Can you work these out from the model? Positions are in its coordinate system, mm. A direction names the side the tool comes from. Round coordinates to 2 decimals unless told otherwise and drop trailing zeros. Loops run counter-clockwise (first coordinate to the right, second up) from the corner with the lowest first, then second, coordinate; pieces in that order, holes last. Notation, with made-up numbers: M 54.5,12.25 L 76.5,12.25 A25 ccw 76.5,25.25 Z; hole C 65,62 d2. An arc over 180 degrees is marked long. Return JSON: item names as keys, results as strings.
```python
from build123d import *

# Parameters (mm, degrees)
SKETCH1_W                       = 254
SKETCH1_H                       = 1016
BOSS_EXTRUDE1_DEPTH             = 203.2
FILLET1_RADIUS                  = 101.6
FILLET1_LENGTH                  = 254
BOSS_EXTRUDE2_DEPTH             = 25.4
BOSS_EXTRUDE2_DEPTH_BACK        = 279.4
SKETCH2_R                       = 12.7
CUT_EXTRUDE1_DEPTH              = 195.834
CUT_EXTRUDE1_DEPTH_BACK         = 440.182
SKETCH4_R                       = 12.7
BOSS_EXTRUDE3_REACH             = 1060.604
SKETCH5_W                       = 660.4
SKETCH5_H                       = 254
BOSS_EXTRUDE3_DIRECTION_2_REACH = 1060.604


with BuildPart() as part:
    # Sketch1 → Boss-Extrude1 (new body)
    with BuildSketch(Plane.XY):
        with Locations((127, 508)):
            Rectangle(SKETCH1_W, SKETCH1_H)
    extrude(amount=BOSS_EXTRUDE1_DEPTH)

    # Fillet1: full round fillet: the end face becomes a half cylinder, R = half its width
    fillet1_face = Plane((127, 0, 101.6), x_dir=(1, 0, 0), z_dir=(0, -1, 0))  # on the end face: x along it, z out of the body
    fillet1_slab = fillet1_face.offset(-FILLET1_RADIUS / 2) * Box(FILLET1_LENGTH, 2 * FILLET1_RADIUS, FILLET1_RADIUS, mode=Mode.PRIVATE)  # the body's end, R deep
    fillet1_round = Plane((127, 101.6, 101.6), x_dir=(0, -1, 0), z_dir=(1, 0, 0)) * Cylinder(FILLET1_RADIUS, FILLET1_LENGTH, mode=Mode.PRIVATE)  # its axis R under the face
    add(fillet1_slab - fillet1_round, mode=Mode.SUBTRACT)

    # Sketch2 → Boss-Extrude2 (add, two sides: drawn at the far end of the back side and taken through both)
    with BuildSketch(Plane(origin=(254, 0, 0), x_dir=(0, 0, -1), z_dir=(1, 0, 0)).offset(-BOSS_EXTRUDE2_DEPTH_BACK)):
        with Locations((-101.6, 25.4)):
            Circle(SKETCH2_R)
    extrude(amount=BOSS_EXTRUDE2_DEPTH + BOSS_EXTRUDE2_DEPTH_BACK)

    # Sketch4 → Cut-Extrude1 (cut, two sides: drawn at the far end of the back side and taken through both)
    with BuildSketch(Plane(origin=(254, 0, 0), x_dir=(0, 0, -1), z_dir=(1, 0, 0)).offset(-CUT_EXTRUDE1_DEPTH_BACK)):
        with Locations(Location((-101.6, 482.6, 0), (0, 0, 180))):
            Circle(SKETCH4_R)
    extrude(amount=CUT_EXTRUDE1_DEPTH + CUT_EXTRUDE1_DEPTH_BACK, mode=Mode.SUBTRACT)

    # Boss-Extrude3: up to this face of the body (flat: up to its plane)
    boss_extrude3_end = Plane(part.part.faces().sort_by_distance((127, 558.8, 203.2))[0])
    # Sketch5 → Boss-Extrude3 (add, up to the picked face)
    with BuildSketch(Plane.XY.offset(101.6), mode=Mode.PRIVATE) as boss_extrude3_sk1:
        with Locations((127, 889)):
            Rectangle(SKETCH5_W, SKETCH5_H)
    boss_extrude3_tool1 = split(extrude(boss_extrude3_sk1.sketch, amount=BOSS_EXTRUDE3_REACH, mode=Mode.PRIVATE), bisect_by=boss_extrude3_end, keep=Keep.BOTH, mode=Mode.PRIVATE)
    add(boss_extrude3_tool1.solids().sort_by(Axis((127, 889, 101.6), (0, 0, 1)))[0])

    # Boss-Extrude3 direction 2: up to this face of the body (flat: up to its plane)
    boss_extrude3_direction_2_end = Plane(part.part.faces().sort_by_distance((127, 558.8, 0))[0])
    # Sketch5 → Boss-Extrude3 direction 2 (add, up to the picked face)
    with BuildSketch(Plane.XY.offset(101.6), mode=Mode.PRIVATE) as boss_extrude3_direction_2_sk1:
        with Locations((127, 889)):
            Rectangle(SKETCH5_W, SKETCH5_H)
    boss_extrude3_direction_2_tool1 = split(extrude(boss_extrude3_direction_2_sk1.sketch, amount=-BOSS_EXTRUDE3_DIRECTION_2_REACH, mode=Mode.PRIVATE), bisect_by=boss_extrude3_direction_2_end, keep=Keep.BOTH, mode=Mode.PRIVATE)
    add(boss_extrude3_direction_2_tool1.solids().sort_by(Axis((127, 889, 101.6), (0, 0, -1)))[0])


solid = part.part
```
Q1. Suppose I cut it at C-C, the plane x = 83. Please give me the cut outline in (y, z), plus the area to 3 significant figures.
Results:
{"outline": "M 101.6,0 L 1016,0 L 1016,203.2 L 101.6,203.2 A101.6 ccw Z; hole C 482.6,101.6 d25.4", "area": "202,000 mm2"}
Q2. Thinking about a two-plate mould opening in Z: for faces 1 (the cylindrical face through (128.778, 0.025, 103.834)), 2 (the flat face through (457.2, 887, 100)), 3 (the cylindrical face through (125.22, 495, 98.85)), 4 (the flat face through (122, 654, 0)), which applies, pulls with the +Z half, pulls with the -Z half, needs draft (parallel to the pull), parting line crosses it, or undercut?
Results:
{"face 1": "parting line crosses it", "face 2": "needs draft", "face 3": "undercut", "face 4": "pulls with the -Z half"}
Q3. On a 3-axis mill with a long thin cutter (end or side, diameter ignored), from which of +Z, -Z, +X, -X, +Y, -Y can I reach the whole of each face in a straight line? I mean faces 5 (the cylindrical face through (266.522, 29.215, 89.486)), 6 (the flat face through (279.4, 26, 102)), 7 (the cylindrical face through (-12.878, 29.215, 89.486)), 8 (the flat face through (-25.4, 26, 102)). Say none if no direction works.
Results:
{"face 5": "+X", "face 6": "+Z, -Z, +X, -Y", "face 7": "-X", "face 8": "+Z, -Z, -X, -Y"}
Q4. If I drill on line 1 along Y through (x, z) = (137.5, 101.6); line 2 along Z through (x, y) = (191, 482); line 3 along X through (y, z) = (300.5, 120), over which ranges is the centre line in solid material (lowest first)?
Results:
{"line 1": "y = 0 to 469.9, 495.3 to 1016", "line 2": "z = 0 to 88.91, 114.29 to 203.2", "line 3": "x = 0 to 254"}
Q5. Suppose I cut it at D-D, the plane z = 48. Please give me the cut outline in (x, y).
Results:
{"outline": "M -203.2,762 L 0,762 L 0,15.29 L 254,15.29 L 254,762 L 457.2,762 L 457.2,1016 L -203.2,1016 Z"}
Q6. Suppose I cut it at B-B, the plane y = 482.6. Please give me the cut outline in (x, z).
Results:
{"outline": "M 0,0 L 254,0 L 254,88.9 L 0,88.9 Z; M 0,114.3 L 254,114.3 L 254,203.2 L 0,203.2 Z"}
Q7. I'm going to push flat-ended pins straight in: pin 1 Ø10 at (y, z) = (643, 118.5) entering from +X; pin 2 Ø3 at (y, z) = (555, 164) entering from -X; pin 3 Ø15 at (y, z) = (482.6, 101.6) entering from -X; pin 4 Ø20.5 at (y, z) = (25.5, 105.5) entering from -X. Where does each tip first touch, or does it pass through?
Results:
{"pin 1": "stops at x = 254", "pin 2": "stops at x = 0", "pin 3": "passes through", "pin 4": "stops at x = -25.4"}
Q8. Suppose I cut it at A-A, the plane z = 101.6. Please give me the cut outline in (x, y).
Results:
{"outline": "M -203.2,762 L 0,762 L 0,495.3 L 254,495.3 L 254,762 L 457.2,762 L 457.2,1016 L -203.2,1016 Z; M -25.4,12.7 L 0,12.7 L 0,0 L 254,0 L 254,12.7 L 279.4,12.7 L 279.4,38.1 L 254,38.1 L 254,469.9 L 0,469.9 L 0,38.1 L -25.4,38.1 Z"}
